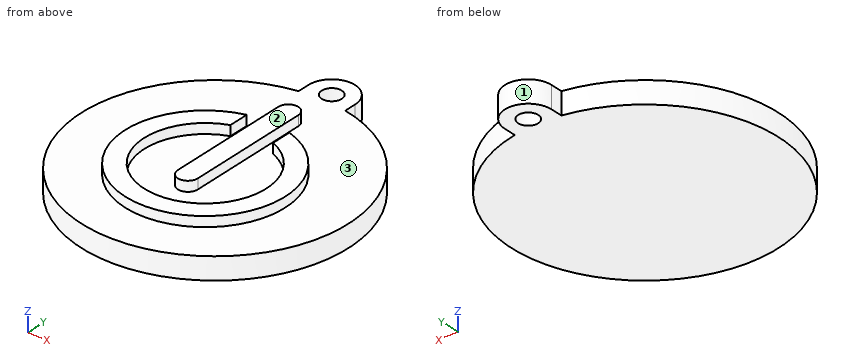
```python
from build123d import *

# Parameters (mm, degrees)
EXTRUDE_DEPTH = 3.3
SKETCH001_R   = 1.5
POCKET_DEPTH  = 3.301
PAD_DEPTH     = 1.5


with BuildPart() as part:
    # Sketch → Extrude (new body)
    with BuildSketch(Plane.XY):
        with BuildLine():
            ThreePointArc((3.5, 21.5), (0, 25), (-3.5, 21.5))
            Line((-3.5, 21.5), (-3.5, 19.691369))
            ThreePointArc((-3.5, 19.691369), (0, -20), (3.5, 19.691369))
            Line((3.5, 19.691369), (3.5, 21.5))
        make_face()
    extrude(amount=EXTRUDE_DEPTH)

    # Sketch001 → Pocket (cut, through all)
    with BuildSketch(Plane.XY.offset(3.3)):
        with Locations((0, 21.5)):
            Circle(SKETCH001_R)
    extrude(amount=-POCKET_DEPTH, mode=Mode.SUBTRACT)

    # Sketch002 → Pad (new body, symmetric)
    with BuildSketch(Plane.XY.offset(3.3)):
        with BuildLine():
            Line((-1.5, 13.5), (-1.5, -5))
            ThreePointArc((-1.5, -5), (0, -6.5), (1.5, -5))
            Line((1.5, -5), (1.5, 13.5))
            ThreePointArc((1.5, 13.5), (0, 15), (-1.5, 13.5))
        make_face()
        with BuildLine():
            ThreePointArc((-3.2, 6.765466), (0, -10.943698), (3.2, 6.765466))
            Line((3.2, 9.765466), (3.2, 6.765466))
            ThreePointArc((-3.2, 9.765466), (0, -13.8), (3.2, 9.765466))
            Line((-3.2, 6.765466), (-3.2, 9.765466))
        make_face()
    extrude(amount=PAD_DEPTH, both=True)


solid = part.part
```
Geometry: final body of the model. Coordinates: model frame, mm. Face numbers are marked on the shaded views. Give positions to 0.01 mm unless a question says otherwise; leave off trailing zeros. Order: outer loops, then holes, each group sorted by start corner. A loop starts at its lowest first (then second) coordinate and runs counter-clockwise, first axis right, second up. Notation, with made-up numbers: (-4.5, -15) -> (11.5, -15) arc R28 ccw to (11.5, 4) -> close; hole circle Ø3 at (72.25, 73.5). An arc over 180 degrees is marked (long way). Write each question's results on one line, items separated by ' | '. Start each with the question number.
1) Section C-C (y = 14). Return loops of the section in (x, z), then the cut area to 3 significant figures.
2) First-contact query: pin 1 (5 mm diameter, centred on x = -15.5, y = -3.5, fed in from +Z); pin 2 (0.5 mm diameter, centred on y = 20, z = 1.5, fed in from -X); pin 3 (0.9 mm diameter, centred on y = 21, z = 2, fed in from +X). Flat tips, straight axial feed; report the tip coordinate or a pass-through.
3) Section D-D (x = 4.5). Return loops of the section in (y, z), then the cut area to 3 significant figures.
4) Section B-B (x = 0). Return loops of the section in (y, z).
5) Draft query along X for the marked faces 1, 2 and 3. Return one class per face: pulls with the +X half, pulls with the -X half, needs draft (parallel to the pull), parting line crosses it, or undercut.
6) Section A-A (z = 4.2). Return loops of the section in (x, y), then the cut area to 3 significant figures.
7) Line query: line 1 (X direction, y = -1.8, z = 4.1); line 2 (X direction, y = 7.5, z = 4.35); line 3 (Y direction, x = 0, z = 0.95). Output: solid intervals per line, ascending. Write a range as from..to.
Calculated:
1) outline: (-14.28, 0) -> (14.28, 0) -> (14.28, 3.3) -> (1.41, 3.3) -> (1.41, 4.8) -> (-1.41, 4.8) -> (-1.41, 3.3) -> (-14.28, 3.3) -> close | area: 98.5 mm2
2) pin 1: z = 3.3 | pin 2: x = -3.5 | pin 3: x = 3.5
3) outline: (-19.49, 0) -> (19.49, 0) -> (19.49, 3.3) -> (9.32, 3.3) -> (9.32, 4.8) -> (6.16, 4.8) -> (6.16, 3.3) -> (-9.76, 3.3) -> (-9.76, 4.8) -> (-12.92, 4.8) -> (-12.92, 3.3) -> (-19.49, 3.3) -> close | area: 138 mm2
4) outline: (-20, 0) -> (20, 0) -> (20, 3.3) -> (15, 3.3) -> (15, 4.8) -> (-6.5, 4.8) -> (-6.5, 3.3) -> (-10.94, 3.3) -> (-10.94, 4.8) -> (-13.8, 4.8) -> (-13.8, 3.3) -> (-20, 3.3) -> close; (23, 0) -> (25, 0) -> (25, 3.3) -> (23, 3.3) -> close
5) face 1: parting line crosses it | face 2: needs draft | face 3: undercut
6) outline: (-3.2, 6.77) -> (-3.2, 9.77) arc R12 ccw (long way) to (3.2, 9.77) -> (3.2, 6.77) arc R9.14 cw (long way) to start; (-1.5, -5) arc R1.5 ccw to (1.5, -5) -> (1.5, 13.5) arc R1.5 ccw to (-1.5, 13.5) -> close | area: 234 mm2
7) line 1: -12..-9.14, -1.5..1.5, 9.14..12 | line 2: -7.58..-3.2, -1.5..1.5, 3.2..7.58 | line 3: -20..20, 23..25
